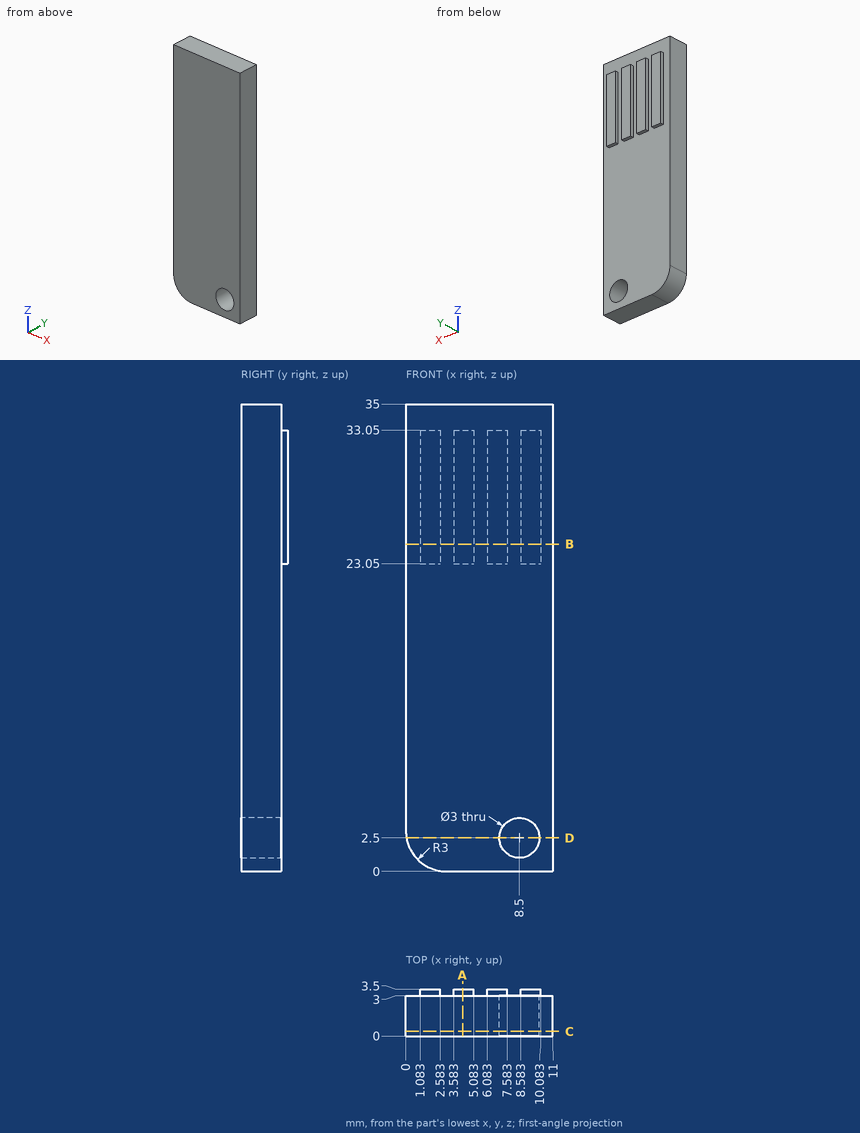
For this review, use the dimensioned drawing (mm, ordinates from the lowest corner) and the shaded views. Round coordinates to 2 decimals unless told otherwise and drop trailing zeros. Write each loop counter-clockwise with the first axis right and the second up, starting at its lowest first coordinate (ties: lowest second). Pieces come first, ordered by that corner, then holes. Notation, with made-up numbers: (59.5, -27) -> (85.5, -27) arc R21 cw to (85.5, 9) -> close; hole circle Ø8 at (2, 79). An arc over 180 degrees is marked (long way). One line per item, written item: value. Start each with the question number.
Q1. Add section B-B (z = 24.5). Give the boundary of the cut face in (x, y).
Q2. Add section C-C (y = 0.35). Give the boundary of the cut face in (x, z), then the cut area to 3 significant figures.
Q3. Add section D-D (z = 2.5). Give the boundary of the cut face in (x, y).
Q4. Add section A-A (x = 4.25). Give the boundary of the cut face in (y, z), then the cut area to 3 significant figures.
Q5. To check wall thickness, follow probe 1 along X at (y, z) = (1.2, 2.5); probe 2 along Z at (x, y) = (9.75, 2.8); probe 3 along X at (y, z) = (1.1, 3) (1 decimal). State the ranges of each line that lie inside material, in increasing order.
Q6. Insertion check: P1, Ø5, axis at x = 8.5, z = 2.5, coming from the +Y side; P2, Ø0.6, axis at y = 3.5, z = 27.5, coming from the +X side; P3, Ø0.6, axis at y = 3, z = 30.5, coming from the -X side. Each pin has a flat end and moves straight along its axis. Give the tip position at first contact, or say it passes through.
Response:
1. outline: (0, 0) -> (11, 0) -> (11, 3) -> (10.08, 3) -> (10.08, 3.5) -> (8.58, 3.5) -> (8.58, 3) -> (7.58, 3) -> (7.58, 3.5) -> (6.08, 3.5) -> (6.08, 3) -> (5.08, 3) -> (5.08, 3.5) -> (3.58, 3.5) -> (3.58, 3) -> (2.58, 3) -> (2.58, 3.5) -> (1.08, 3.5) -> (1.08, 3) -> (0, 3) -> close
2. outline: (0, 3) arc R3 ccw to (3, 0) -> (11, 0) -> (11, 35) -> (0, 35) -> close; hole circle Ø3 at (8.5, 2.5)
2. area: 376 mm^2
3. outline: (0.04, 0) -> (7, 0) -> (7, 3) -> (0.04, 3) -> close; (10, 0) -> (11, 0) -> (11, 3) -> (10, 3) -> close
4. outline: (0, 0) -> (3, 0) -> (3, 23.05) -> (3.5, 23.05) -> (3.5, 33.05) -> (3, 33.05) -> (3, 35) -> (0, 35) -> close
4. area: 110 mm^2
5. probe 1: x = 0.04 to 7, 10 to 11
5. probe 2: z = 0 to 1.67, 3.33 to 35
5. probe 3: x = 0 to 7.1, 9.9 to 11
6. P1: stops at y = 3
6. P2: stops at x = 10.08
6. P3: stops at x = 0
